Geometry check sheet. Reference: the model listing, model coordinates, mm. A direction names the side the tool comes from. Give positions to 0.01 mm unless a question says otherwise; leave off trailing zeros. Order: outer loops, then holes, each group sorted by start corner. A loop starts at its lowest first (then second) coordinate and runs counter-clockwise, first axis right, second up.
from build123d import *

# Parameters (mm, degrees)
SKETCH2_W      = 2
SKETCH2_H      = 9.797583912
EXTRUDE1_DEPTH = 1


with BuildPart() as part:
    # Sketch1 → Revolve1 (revolve)
    with BuildSketch(Plane.XY, mode=Mode.PRIVATE) as revolve1_sk:
        Polygon((0, 0), (-4.5, 0), (-3, -1.5), (-3, -17.5), (0, -19.232050808), (0, -17.5), align=None)
    revolve(revolve1_sk.sketch.rotate(Axis((0, 0, 0), (0, -1, 0)), 270), axis=Axis((0, 0, 0), (0, -1, 0)))

    # Sketch2 → Extrude1 (cut)
    with BuildSketch(Plane(origin=(0, 0, 0), x_dir=(1, 0, 0), z_dir=(0, 1, 0))):
        with Locations((0, -0.007322559)):
            Rectangle(SKETCH2_W, SKETCH2_H)
    extrude(amount=-EXTRUDE1_DEPTH, mode=Mode.SUBTRACT)


solid = part.part
Item 1: Set-up check for faces 1 (the flat face through (-1, -0.5, 0.1)), 2 (the flat face through (-2, 0, 0)), 3 (the cylindrical face through (-0.9, -9.61, 2.86)): record each of +Z, -Z, +X, -X, +Y, -Y from which the full face is reachable in a straight line by a thin tool's end or side.
Reported:
face 1: +Z, -Z, +Y
face 2: +Z, -Z, +X, -X, +Y
face 3: -Y
Item 2: Sectioned sample at A-A (y = -10). Enter the section's corners in (x, z).
Reported:
outline: circle Ø6 at (0, 0)
Item 3: Sectioned sample at B-B (y = -18). Enter the section's corners in (x, z).
Reported:
outline: circle Ø4.27 at (0, 0)
Item 4: Gauge pin test, flat ends, axial feed: pin 1 (3 mm diameter, centred on x = 3.5, z = 0, fed in from -Y); pin 2 (1 mm diameter, centred on x = -2, y = -4.5, fed in from -Z); pin 3 (4 mm diameter, centred on y = -8, z = 3.5, fed in from -X). Record the tip position at first contact, or that the pin passes through.
Reported:
pin 1: stops at y = -18.08
pin 2: stops at z = -2.6
pin 3: stops at x = -2.6
Item 5: Scan lines: L1, parallel to X at y = -11.25, z = 0; L2, parallel to Z at x = -2.75, y = -9.5; L3, parallel to Z at x = 0.5, y = -14.5. Record each from-to range of solid material in increasing order.
Reported:
L1: x = -3 to 3
L2: z = -1.2 to 1.2
L3: z = -2.96 to 2.96
